```python
from build123d import *

# Parameters (mm, degrees)
SKETCH1_W           = 200
SKETCH1_H           = 70
SKETCH1_R           = 2.65
SKETCH1_R_2         = 8.5
BOSS_EXTRUDE1_DEPTH = 3


with BuildPart() as part:
    # Sketch1 → Boss-Extrude1 (new body)
    with BuildSketch(Plane.YZ):
        Rectangle(SKETCH1_W, SKETCH1_H)
        with Locations(Location((-76, -15.6, 0), (0, 0, 270))):
            Circle(SKETCH1_R, mode=Mode.SUBTRACT)
        with Locations(Location((76, -15.6, 0), (0, 0, 90))):
            Circle(SKETCH1_R, mode=Mode.SUBTRACT)
        with Locations(Location((-70, 15, 0), (0, 0, 270))):
            Circle(SKETCH1_R, mode=Mode.SUBTRACT)
        with Locations(Location((70, 15, 0), (0, 0, 90))):
            Circle(SKETCH1_R, mode=Mode.SUBTRACT)
        with Locations(Location((0, 0, 0), (0, 0, 270))):
            Circle(SKETCH1_R_2, mode=Mode.SUBTRACT)
    extrude(amount=BOSS_EXTRUDE1_DEPTH)


solid = part.part
```
Build history of the part. All positions in model axes, mm. Coordinates: 2 decimals unless noted, no trailing zeros. Order: outer loops, then holes, each group sorted by start corner. A loop starts at its lowest first (then second) coordinate and runs counter-clockwise, first axis right, second up.
Item 1: Mould opens along Y. For faces 1 (the cylindrical face through (1.48, 78.59, -16.17)), 2 (the flat face through (3, -1, -15)), 3 (the cylindrical face through (1.479, -72.351, 13.777)) say: released by +Y, released by -Y, zero draft, split by the parting line, or undercut.
Filled in:
face 1: undercut
face 2: zero draft
face 3: undercut
Item 2: Saw through at D-D on z = -3. List the corners of the cut face in (x, y), then the cut area to 3 significant figures.
Filled in:
outline: (0, -100) - (3, -100) - (3, -7.95) - (0, -7.95) - close; (0, 7.95) - (3, 7.95) - (3, 100) - (0, 100) - close
area: 552 mm2
Item 3: Saw through at B-B on z = -15.6. List the corners of the cut face in (x, y), then the cut area to 3 significant figures.
Filled in:
outline: (0, -100) - (3, -100) - (3, -78.65) - (0, -78.65) - close; (0, -73.35) - (3, -73.35) - (3, 73.35) - (0, 73.35) - close; (0, 78.65) - (3, 78.65) - (3, 100) - (0, 100) - close
area: 568 mm2
Item 4: Saw through at A-A on y = 70. List the corners of the cut face in (x, z).
Filled in:
outline: (0, -35) - (3, -35) - (3, 12.35) - (0, 12.35) - close; (0, 17.65) - (3, 17.65) - (3, 35) - (0, 35) - close
Item 5: Drill centre lines: L1, parallel to Y at x = 0.7, z = 15; L2, parallel to Y at x = 1.8, z = 16; L3, parallel to Y at x = 1.35, z = 0. Where is each one in solid material? Low to high.
Filled in:
L1: y = -100 to -72.65, -67.35 to 67.35, 72.65 to 100
L2: y = -100 to -72.45, -67.55 to 67.55, 72.45 to 100
L3: y = -100 to -8.5, 8.5 to 100
Item 6: Saw through at C-C on x = 1.6. List the corners of the cut face in (y, z), then the cut area to 3 significant figures.
Filled in:
outline: (-100, -35) - (100, -35) - (100, 35) - (-100, 35) - close; hole circle Ø5.3 at (-76, -15.6); hole circle Ø5.3 at (-70, 15); hole circle Ø17 at (0, 0); hole circle Ø5.3 at (70, 15); hole circle Ø5.3 at (76, -15.6)
area: 13,700 mm2
